Model file for the job. Use its own axes, mm. A direction names the side the tool comes from. Coordinates: 2 decimals unless noted, no trailing zeros. Order: outer loops, then holes, each group sorted by start corner. A loop starts at its lowest first (then second) coordinate and runs counter-clockwise, first axis right, second up. Notation, with made-up numbers: (33.25, 17.5) -> (48.25, 17.5) arc R25 ccw to (48.25, 31.5) -> close; hole circle Ø10 at (57, -32.5). An arc over 180 degrees is marked (long way). Return JSON: item names as keys, results as strings. Group by question number.
1) Cut at A-A (y = -4.25). Write the cut outline in (x, z), and give its area (3 significant figures).
2) Cut at D-D (z = -24.13). Write the cut outline in (x, y), and give its area (3 significant figures).
3) Cut at C-C (x = 80.4). Write the cut outline in (y, z).
4) Probe line 1 (Z direction, x = 80.4, y = -5.25); line 2 (X direction, y = 6.4, z = -24.13); line 3 (X direction, y = 2.75, z = -24.13). List the from-to ranges inside material, lowest first.
5) Pull direction X, two halves, no side cores. Call faces 4 (the cylindrical face through (31.95, 4.51, -15.48)), 5 (the cylindrical face through (27.443, -3.863, -0.764)), 6 (the flat face through (31, -4, -23.241)), 7 (the cylindrical face through (84.25, -3.86, -0.78)): +X half, -X half, draft (parallel to the pull), parting line (faces both ways), or undercut.
6) Which spindle directions (+Z, -Z, +X, -X, +Y, -Y) get a long thin tool onto all of the face, cutting with end or side? Do faces 1 (the flat face through (80, -4, -23.241)), 2 (the flat face through (56, -7.62, -2)), 3 (the cylindrical face through (96.77, 1.88, -24.38)). Say none if no direction does.
7) Flat gauge pins, fed straight in: pin 1 (12.5 mm diameter, centred on x = 12.5, z = -21.5, fed in from -Y); pin 2 (8.5 mm diameter, centred on x = 91.059, z = -24.13, fed in from -Y); pin 3 (3 mm diameter, centred on x = 48.5, y = -5.5, fed in from -Z). Where does each tip first touch, or does it go through?
8) Cut at B-B (x = 55). Write the cut outline in (y, z), and give its area (3 significant figures).
from build123d import *

# Parameters (mm, degrees)
SKETCH1_W             = 101.6
SKETCH1_H             = 35.052
INITIAL_EXTRUDE_DEPTH = 8.89
SKETCH2_R             = 3.302
SCREW_HOLES_DEPTH     = 9.89
SKETCH4_R             = 2.5
SKETCH4_W             = 40.432286119
SKETCH4_H             = 21.082
SERVO_HOLE_DEPTH      = 9.89
FILLET1_R             = 6.35
SKETCH6_R             = 5.715
SCREW_HEAD_HOLE_DEPTH = 3.81
SKETCH7_W             = 8.89
SKETCH7_H             = 21.082
SKETCH7_R             = 2.55
BOSS_EXTRUDE1_DEPTH   = 7.62
FILLET2_R             = 2.54
BOSS_EXTRUDE2_DEPTH   = 7.62
FILLET3_R             = 2.54


with BuildPart() as part:
    # Sketch1 → Initial Extrude (new body)
    with BuildSketch(Plane(origin=(0, 0, 0), x_dir=(1, 0, 0), z_dir=(0, 1, 0))):
        with Locations((50.8, 17.526)):
            Rectangle(SKETCH1_W, SKETCH1_H)
    extrude(amount=INITIAL_EXTRUDE_DEPTH)

    # Sketch2 → Screw Holes (cut, through all)
    with BuildSketch(Plane(origin=(0, 8.89, 0), x_dir=(1, 0, 0), z_dir=(0, 1, 0))):
        with Locations((10.541, 8.89)):
            Circle(SKETCH2_R)
        with Locations((91.059, 24.13)):
            Circle(SKETCH2_R)
        with Locations((10.541, 24.13)):
            Circle(SKETCH2_R)
        with Locations((91.059, 8.89)):
            Circle(SKETCH2_R)
    extrude(amount=-SCREW_HOLES_DEPTH, mode=Mode.SUBTRACT)

    # Sketch4 → Servo Hole (cut, through all)
    with BuildSketch(Plane(origin=(0, 8.89, 0), x_dir=(1, 0, 0), z_dir=(0, 1, 0))):
        with Locations((30.8, 7.7)):
            Circle(SKETCH4_R)
        with Locations((30.8, 17.7)):
            Circle(SKETCH4_R)
        with Locations((55.824856941, 12.7)):
            Rectangle(SKETCH4_W, SKETCH4_H)
        with Locations((80.4, 17.7)):
            Circle(SKETCH4_R)
        with Locations((80.4, 7.7)):
            Circle(SKETCH4_R)
    extrude(amount=-SERVO_HOLE_DEPTH, mode=Mode.SUBTRACT)

    # Fillet1
    fillet1_edges = [part.edges().sort_by_distance(p)[0] for p in [
        (0, 4.445, 0),
        (0, 4.445, -35.052),
        (101.6, 4.445, -35.052),
        (101.6, 4.445, 0),
    ]]
    fillet(fillet1_edges, radius=FILLET1_R)

    # Sketch6 → Screw Head Hole (cut)
    with BuildSketch(Plane(origin=(0, 0, 0), x_dir=(-1, 0, 0), z_dir=(0, -1, 0))):
        with Locations((-10.541, 8.89)):
            Circle(SKETCH6_R)
        with Locations((-10.541, 24.13)):
            Circle(SKETCH6_R)
        with Locations((-91.059, 24.13)):
            Circle(SKETCH6_R)
        with Locations((-91.059, 8.89)):
            Circle(SKETCH6_R)
    extrude(amount=-SCREW_HEAD_HOLE_DEPTH, mode=Mode.SUBTRACT)

    # Sketch7 → Boss-Extrude1 (add)
    with BuildSketch(Plane.XZ):
        with Locations((31.163713881, -12.7)):
            Rectangle(SKETCH7_W, SKETCH7_H)
        with Locations((30.8, -7.7)):
            Circle(SKETCH7_R, mode=Mode.SUBTRACT)
        with Locations((30.8, -17.7)):
            Circle(SKETCH7_R, mode=Mode.SUBTRACT)
        with Locations((80.486, -12.7)):
            Rectangle(SKETCH7_W, SKETCH7_H)
        with Locations((80.4, -7.7)):
            Circle(SKETCH7_R, mode=Mode.SUBTRACT)
        with Locations((80.4, -17.7)):
            Circle(SKETCH7_R, mode=Mode.SUBTRACT)
    extrude(amount=BOSS_EXTRUDE1_DEPTH)

    # Fillet2
    fillet2_edges = [part.edges().sort_by_distance(p)[0] for p in [
        (35.608713881, -3.81, -23.241),
        (35.608713881, -3.81, -2.159),
        (26.718713881, -3.81, -2.159),
        (26.718713881, -3.81, -23.241),
        (76.041, -3.81, -2.159),
        (76.041, -3.81, -23.241),
        (84.931, -3.81, -23.241),
        (84.931, -3.81, -2.159),
    ]]
    fillet(fillet2_edges, radius=FILLET2_R)

    # Sketch8 → Boss-Extrude2 (add)
    with BuildSketch(Plane.XZ):
        Polygon((26.718713881, -4.699), (26.718713881, 0), (84.997322511, 0), (84.931, -4.699), (76.041, -4.699), (76.041, -2.159), (35.608713881, -2.159), (35.608713881, -4.699), align=None)
    extrude(amount=BOSS_EXTRUDE2_DEPTH)

    # Fillet3
    fillet3_edges = [part.edges().sort_by_distance(p)[0] for p in [
        (26.718713881, -3.81, 0),
        (84.997322511, -3.81, 0),
        (76.041, 0.635, -2.159),
        (35.608713881, 0.635, -2.159),
    ]]
    fillet(fillet3_edges, radius=FILLET3_R)


solid = part.part
Answers below:
{
 "1": {"outline": "(26.72, -20.7) arc R2.54 ccw to (29.26, -23.24) -> (33.07, -23.24) arc R2.54 ccw to (35.61, -20.7) -> (35.61, -4.7) arc R2.54 cw to (38.15, -2.16) -> (73.5, -2.16) arc R2.54 cw to (76.04, -4.7) -> (76.04, -20.7) arc R2.54 ccw to (78.58, -23.24) -> (82.39, -23.24) arc R2.54 ccw to (84.93, -20.7) -> (84.93, -4.7) -> (84.96, -2.58) arc R2.54 ccw to (82.42, 0) -> (29.26, 0) arc R2.54 ccw to (26.72, -2.54) -> close; hole circle Ø5.1 at (30.8, -17.7); hole circle Ø5.1 at (30.8, -7.7); hole circle Ø5.1 at (80.4, -17.7); hole circle Ø5.1 at (80.4, -7.7)", "area": "413 mm^2"},
 "2": {"outline": "(0, 0) -> (4.83, 0) -> (4.83, 3.81) -> (7.24, 3.81) -> (7.24, 8.89) -> (0, 8.89) -> close; (13.84, 3.81) -> (16.26, 3.81) -> (16.26, 0) -> (85.34, 0) -> (85.34, 3.81) -> (87.76, 3.81) -> (87.76, 8.89) -> (13.84, 8.89) -> close; (94.36, 3.81) -> (96.77, 3.81) -> (96.77, 0) -> (101.6, 0) -> (101.6, 8.89) -> (94.36, 8.89) -> close", "area": "749 mm^2"},
 "3": {"outline": "(-7.62, -23.24) -> (0, -23.24) -> (0, -35.05) -> (8.89, -35.05) -> (8.89, -20.2) -> (0, -20.2) -> (0, -20.25) -> (-7.62, -20.25) -> close; (-7.62, -15.15) -> (0, -15.15) -> (0, -15.2) -> (8.89, -15.2) -> (8.89, -10.2) -> (0, -10.2) -> (0, -10.25) -> (-7.62, -10.25) -> close; (-7.62, -5.15) -> (0, -5.15) -> (0, -5.2) -> (8.89, -5.2) -> (8.89, 0) -> (-7.62, 0) -> close"},
 "4": {"line 1": "z = -23.24 to -20.25, -15.15 to -10.25, -5.15 to 0", "line 2": "x = 0 to 7.24, 13.84 to 87.76, 94.36 to 101.6", "line 3": "x = 0 to 4.83, 16.26 to 85.34, 96.77 to 101.6"},
 "5": {"face 4": "undercut", "face 5": "-X half", "face 6": "draft", "face 7": "+X half"},
 "6": {"face 1": "-Z, +X, -X, -Y", "face 2": "+Z, -Z, +X, -X, -Y", "face 3": "-Y"},
 "7": {"pin 1": "stops at y = 0", "pin 2": "stops at y = 3.81", "pin 3": "stops at z = -2.16"},
 "8": {"outline": "(-7.62, -2.16) -> (8.89, -2.16) -> (8.89, 0) -> (-7.62, 0) -> close; (0, -35.05) -> (8.89, -35.05) -> (8.89, -23.24) -> (0, -23.24) -> close", "area": "141 mm^2"}
}
